The listing builds one solid part. Answer for the finished solid, in the listing's coordinates (mm). Face numbers are marked on the shaded views. A direction names the side the tool comes from. Give positions to 0.01 mm unless a question says otherwise; leave off trailing zeros. Loops run counter-clockwise (first coordinate to the right, second up) from the corner with the lowest first, then second, coordinate; pieces in that order, holes last. Notation, with made-up numbers: (71.25, -7.5) - (125.25, -7.5) arc R21 cw to (125.25, 0.5) - close; hole circle Ø4 at (-20.5, 47). An arc over 180 degrees is marked (long way). Write item = value, one per line. Start each with the question number.
1) Which of the six approach directions +Z, -Z, +X, -X, +Y, -Y give full straight-line access (tool end or side, diameter ignored) to the marked faces 1, 2, 3 and 4?
2) Flat-ended cylindrical pins translate along their axes: P1, Ø3, axis at x = 11, z = -5.5, coming from the -Y side; P2, Ø1, axis at x = 7.5, z = 0.5, coming from the -Y side; P3, Ø1.5, axis at y = 4.5, z = 6, coming from the -X side; P4, Ø0.8, axis at y = -1, z = 5.5, coming from the -X side. Find the tip coordinate at first contact, or state that the pin passes through.
3) Consider probe 1 along Z at (x, y) = (16, 0); probe 2 along Y at (x, z) = (17.75, 0); probe 3 along Z at (x, y) = (2.75, 0). Determine where each line is inside the solid, lowest interval first.
4) The part is cut by section B-B on x = 3.5. Write down the section's boundary in (y, z).
5) The mould has two halves that part along Z. Classify the marked faces 5, 6, 7 and 8: +Z half, -Z half, draft (parallel to the pull), parting line (faces both ways), or undercut.
6) The part is cut by section A-A on x = 22. Write down the section's boundary in (y, z).
from build123d import *

# Parameters (mm, degrees)
F0_W           = 25.4
F0_H           = 2.7813
F2_W           = 1.9558
F2_H           = 1.4605
F4_W           = 13.6652
F4_H           = 2.921
F6_W           = 2.159
F6_H           = 3.2766
F6_W_2         = 2.413
F6_H_2         = 4.572
F8_R           = 3.6576
F9_DEPTH       = 10.541
F10_R          = 4.191
F11_DEPTH      = 3.9624
F12_W          = 4.1148
F12_H          = 3.937
F13_DEPTH      = 7.8115
F13_DEPTH_BACK = 7.8115
F14_SIZE       = 0.254
F15_SIZE       = 0.254
F16_R          = 0.254


# Not quite as in the source:
# - a feature of the source that left no trace in its solid (it failed there, or was rolled back) is left out


with BuildPart() as f1:
    # F0 (on Front) → F1 (revolve)
    with BuildSketch(Plane.XZ):
        with Locations((12.7, 4.95935)):
            Rectangle(F0_W, F0_H)
    revolve(axis=Axis((6.9021734883, 0, 0), (1, 0, 0)))

    # F2 (on Front) → F3 (revolve)
    with BuildSketch(Plane.XZ):
        with Locations((10.7569, 7.08025)):
            Rectangle(F2_W, F2_H)
    revolve(axis=Axis((12.3426117934, 0, 0), (1, 0, 0)))

    # F4 (on Front) → F5 (revolve, cut)
    with BuildSketch(Plane.XZ):
        with Locations((18.5674, 7.4295)):
            Rectangle(F4_W, F4_H)
    revolve(axis=Axis((16.2136404502, 0, 0), (1, 0, 0)), mode=Mode.SUBTRACT)

    # F6 (on Front) → F7 (revolve, cut)
    with BuildSketch(Plane.XZ):
        with Locations((8.6995, 7.2517)):
            Rectangle(F6_W, F6_H)
        with Locations((24.1935, 6.604)):
            Rectangle(F6_W_2, F6_H_2)
    revolve(axis=Axis((7.4812129023, 0, 0), (1, 0, 0)), mode=Mode.SUBTRACT)

    # F8 (on face) → F9 (cut)
    with BuildSketch(Plane(origin=(0, 0, 0), x_dir=(0, -1, 0), z_dir=(-1, 0, 0))):
        Circle(F8_R)
    extrude(amount=-F9_DEPTH, mode=Mode.SUBTRACT)

    # F10 (on face) → F11 (cut)
    with BuildSketch(Plane.YZ.offset(25.4)):
        Circle(F10_R)
    extrude(amount=-F11_DEPTH, mode=Mode.SUBTRACT)

    # F12 (on Front) → F13 (cut, two sides)
    with BuildSketch(Plane.XZ) as f13_sk:
        with Locations((16.9926, 6.9215)):
            Rectangle(F12_W, F12_H)
        with Locations((16.9926, -6.9215)):
            Rectangle(F12_W, F12_H)
    extrude(amount=-F13_DEPTH, mode=Mode.SUBTRACT)
    extrude(f13_sk.sketch, amount=F13_DEPTH_BACK, mode=Mode.SUBTRACT)

    # F14
    f14_edges = [f1.edges().sort_by_distance(p)[0] for p in [
        (9.779, 0, -7.8105),
        (11.7348, 0, -7.8105),
    ]]
    chamfer(f14_edges, length=F14_SIZE)

    # F15
    f15_edges = [f1.edges().sort_by_distance(p)[0] for p in [
        (22.987, 0, -5.969),
    ]]
    chamfer(f15_edges, length=F15_SIZE)

    # F16
    f16_edges = [f1.edges().sort_by_distance(p)[0] for p in [
        (9.779, 0, -5.6134),
        (11.7348, 0, -5.969),
        (22.987, 0, -4.318),
        (21.4376, -4.191, 0),
    ]]
    fillet(f16_edges, radius=F16_R)


solid = f1.part
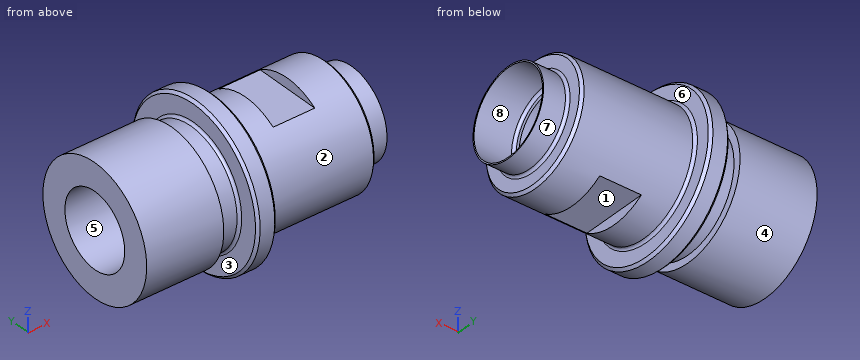
Answer below:
q1.face_1 = -Z, +Y, -Y
q1.face_2 = +X
q1.face_3 = none
q1.face_4 = -X
q2.P1 = -6.71
q2.P2 = -6.35
q2.P3 = 9.78
q2.P4 = 0
q3.probe_1 = -4.95 to -3.57, 3.57 to 4.95
q3.probe_2 = -5.97 to -3.57, 3.57 to 5.97
q3.probe_3 = -6.35 to -3.66, 3.66 to 6.35
q4.outline = circle Ø12.7 at (0, 0); hole circle Ø7.32 at (0, 0)
q5.face_5 = undercut
q5.face_6 = draft
q5.face_7 = parting line
q5.face_8 = undercut
q6.outline = circle Ø11.94 at (0, 0); hole circle Ø8.38 at (0, 0)
